Input: part model. Units: mm. Frame: model coordinates. A direction names the side the tool comes from. Give positions to 0.01 mm unless a question says otherwise; leave off trailing zeros. Loops run counter-clockwise (first coordinate to the right, second up) from the corner with the lowest first, then second, coordinate; pieces in that order, holes last. Notation, with made-up numbers: M 38.5,61 L 64.5,61 A26 cw 64.5,86 Z; hole C -25,5 d6. An arc over 180 degrees is marked long. Use CSV: the item, a comma, the result in double quotes. Start each with the question number.
Autodesk Inventor part; units mm, degrees
ref_plane "YZ Plane" through (0, 0, 0) normal (1, 0, 0) x (0, 1, 0)
ref_plane "XZ Plane" through (0, 0, 0) normal (0, 1, 0) x (-1, 0, 0)
ref_plane "XY Plane" through (0, 0, 0) normal (0, 0, 1) x (1, 0, 0)
sketch "スケッチ1" plane through (0, 0, 0) normal (0, 0, 1) x (1, 0, 0)
  line L0 (-25, 5) -> (25, 5)
  line L1 (25, 5) -> (25, -5)
  line L2 (-25, -5) -> (-25, 5)
  line L3 (-23, 3) -> (23, 3)
  line L4 (23, 3) -> (23, -5)
  line L5 (-23, -5) -> (-23, 3)
  line L6 (25, -5) -> (23, -5)
  line L7 (-23, -5) -> (-25, -5)
  point P0 (0, 0)
  dimension "d0" = 50
  dimension "d2" = 46
  dimension "d3" = 23
  dimension "d4" = 25
  dimension "d5" = 10
  dimension "d6" = 10
  dimension "d8" = 5
  dimension "d9" = 8
extrude "押し出し1" add sketch "スケッチ1" against normal blind 20
sketch "スケッチ2" plane through (25, -5, 0) normal (1, 0, 0) x (0, 0, -1)
  line L0 (0, 10) -> (0, 0)
  line L1 (0, 10) -> (20, 10)
  circle A0 centre (5, 5) radius 1
  circle A1 centre (15, 5) radius 1
  point P0 (0, 5)
  dimension "d14" = 5
  dimension "d15" = 5
  dimension "d16" = 5
  dimension "d17" = 10
  dimension "d18" = 2
hole "穴1" at (25, 0, -5) at (25, 0, -15) direction (-1, 0, 0) diameter 2 end through all
thread "ねじ3"
thread "ねじ4"
thread "ねじ5"
thread "ねじ6"
properties part number "Leg_Link_Conecter" material "アルミニウム 6061"
Item 1: Material intervals for line 1 (Z direction, x = -23.65, y = 0); line 2 (X direction, y = -0.25, z = -18); line 3 (Y direction, x = -23.65, z = -15), sorted ascending.
Item 2: Mould query, pull axis X, two halves, no side actions, for faces 1 (the cylindrical face through (24, 0.6, -4.2)), 2 (the flat face through (25, 0, -10)), 3 (the flat face through (-23, -1, -10)). Classes: +X half, -X half, draft (parallel to the pull), parting line (faces both ways), or undercut.
Item 3: First-contact query: pin 1 Ø1.2 at (y, z) = (0, -5) entering from -X; pin 2 Ø1 at (x, z) = (14, -11) entering from -Y. Flat tips, straight axial feed; report the tip coordinate or a pass-through.
Item 4: Section B-B (y = 0). Output: boundary loops of the cut face in (x, z).
Item 5: Section D-D (x = 1). Output: boundary loops of the cut face in (y, z).
Item 6: Section A-A (z = -15). Output: boundary loops of the cut face in (x, y).
Item 7: Section C-C (y = -4). Output: boundary loops of the cut face in (x, z), then the cut area to 3 significant figures.
Item 8: Set-up query: faces 4 (the cylindrical face through (-24, 0.6, -4.2)), 5 (the flat face through (23, -1, -10)). Return all of +Z, -Z, +X, -X, +Y, -Y with unobstructed straight access to the full face (end or side cutting, diameter ignored); none if empty.
Recorded:
1,line 1,"-20 to -16, -14 to -6, -4 to 0"
1,line 2,"-25 to -23, 23 to 25"
1,line 3,"-5 to -1, 1 to 5"
2,face 1,"draft"
2,face 2,"+X half"
2,face 3,"undercut"
3,pin 1,"through"
3,pin 2,"y = 3"
4,outline,"M -25,-20 L -23,-20 L -23,-16 L -25,-16 Z; M -25,-14 L -23,-14 L -23,-6 L -25,-6 Z; M -25,-4 L -23,-4 L -23,0 L -25,0 Z; M 23,-20 L 25,-20 L 25,-16 L 23,-16 Z; M 23,-14 L 25,-14 L 25,-6 L 23,-6 Z; M 23,-4 L 25,-4 L 25,0 L 23,0 Z"
5,outline,"M 3,-20 L 5,-20 L 5,0 L 3,0 Z"
6,outline,"M -25,-5 L -23,-5 L -23,-1 L -25,-1 Z; M -25,1 L -23,1 L -23,3 L 23,3 L 23,1 L 25,1 L 25,5 L -25,5 Z; M 23,-5 L 25,-5 L 25,-1 L 23,-1 Z"
7,outline,"M -25,-20 L -23,-20 L -23,0 L -25,0 Z; M 23,-20 L 25,-20 L 25,0 L 23,0 Z"
7,area,"80.0 mm²"
8,face 4,"+X, -X"
8,face 5,"+Z, -Z, -Y"
